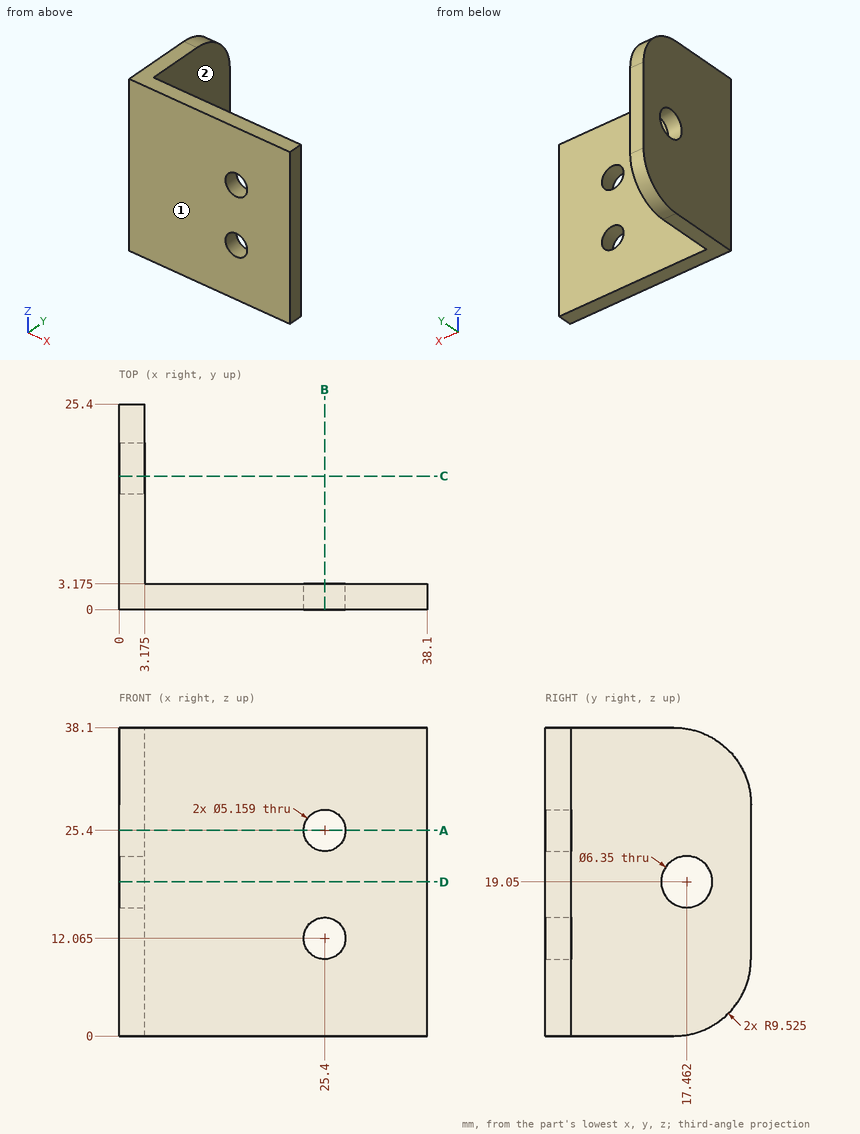
Check sheet for the drawn part. Datum: minimum x, y, z corner. Units: mm. A direction names the side the tool comes from. Coordinates: 2 decimals unless noted, no trailing zeros. Loops run counter-clockwise (first coordinate to the right, second up) from the corner with the lowest first, then second, coordinate; pieces in that order, holes last. Notation, with made-up numbers: (33, 77) -> (86, 77) arc R27 ccw to (86, 94) -> close; hole circle Ø8 at (-27.75, -29.5). An arc over 180 degrees is marked (long way). Answer as a JSON object with one key per item and string values. Group by question number.
Item 1: Sectioned sample at C-C on y = 16.5. Record the boundary of the cut face in (x, z) (1 decimal), plus the area to 3 significant figures.
Item 2: Sectioned sample at A-A on z = 25.4. Record the boundary of the cut face in (x, y) (1 decimal), plus the area to 3 significant figures.
Item 3: Scan lines: probe 1 along Z at (x, y) = (25.4, 2.5) (1 decimal); probe 2 along X at (y, z) = (0.8, 25.4); probe 3 along X at (y, z) = (10, 2.5) (1 decimal). Record each from-to range of solid material in increasing order.
Item 4: Sectioned sample at D-D on z = 19.05. Record the boundary of the cut face in (x, y) (1 decimal).
Item 5: Tool access check on the marked faces 1 and 2. Record the directions out of +Z, -Z, +X, -X, +Y, -Y that give a thin tool (end or side, any length) a straight path to the whole face; none if there is none.
Item 6: Sectioned sample at B-B on x = 25.4. Record the boundary of the cut face in (y, z) (1 decimal).
Item 7: Depth check by flat-ended pin: pin 1 (17.5 mm diameter, centred on x = 18, z = 23, fed in from +Y) (1 decimal); pin 2 (8 mm diameter, centred on y = 18, z = 20, fed in from -X); pin 3 (6.5 mm diameter, centred on y = 9, z = 13, fed in from +X) (1 decimal). Enter the tip coordinate at first touch or a pass-through.
Evaluation:
{
 "1": {"outline": "(0, 0) -> (3.2, 0) -> (3.2, 16) -> (0, 16) -> close; (0, 22.1) -> (3.2, 22.1) -> (3.2, 38.1) -> (0, 38.1) -> close", "area": "102 mm²"},
 "2": {"outline": "(0, 0) -> (22.8, 0) -> (22.8, 3.2) -> (3.2, 3.2) -> (3.2, 25.4) -> (0, 25.4) -> close; (28, 0) -> (38.1, 0) -> (38.1, 3.2) -> (28, 3.2) -> close", "area": "175 mm²"},
 "3": {"probe 1": "z = 0 to 9.5, 14.6 to 22.8, 28 to 38.1", "probe 2": "x = 0 to 22.82, 27.98 to 38.1", "probe 3": "x = 0 to 3.2"},
 "4": {"outline": "(0, 0) -> (38.1, 0) -> (38.1, 3.2) -> (3.2, 3.2) -> (3.2, 14.3) -> (0, 14.3) -> close; (0, 20.6) -> (3.2, 20.6) -> (3.2, 25.4) -> (0, 25.4) -> close"},
 "5": {"face 1": "+Z, -Z, +X, -X, -Y", "face 2": "+Z, -Z, +X, +Y"},
 "6": {"outline": "(0, 0) -> (3.2, 0) -> (3.2, 9.5) -> (0, 9.5) -> close; (0, 14.6) -> (3.2, 14.6) -> (3.2, 22.8) -> (0, 22.8) -> close; (0, 28) -> (3.2, 28) -> (3.2, 38.1) -> (0, 38.1) -> close"},
 "7": {"pin 1": "stops at y = 3.2", "pin 2": "stops at x = 0", "pin 3": "stops at x = 3.2"}
}
